Here's the drawing with two shaded views (mm, measured from the low corner). I have some questions. Coordinates: 2 decimals unless noted, no trailing zeros. Order: outer loops, then holes, each group sorted by start corner. A loop starts at its lowest first (then second) coordinate and runs counter-clockwise, first axis right, second up. Notation, with made-up numbers: (-8, -4) - (33, -4) arc R10 ccw to (33, 8) - close; hole circle Ø5 at (86.25, 27.5). An arc over 180 degrees is marked (long way). Answer as a JSON object with one key per item and string values. Group by question number.
(1) Will this pin go through, and if not, where does the flat tip stop? P1, Ø6.5, axis at x = 7.65, z = 8.87, coming from the -Y side.
(2) Imagine slicing it at A-A, the plane x = 5.5. Write out the boundary of the cut face in (y, z), and give its area (3 significant figures).
(3) Please list where these lines run through material, in increasing order: probe 1 along X at (y, z) = (11.25, 8.5); probe 2 along Z at (x, y) = (56, 10.25); probe 3 along Z at (x, y) = (7, 9.75).
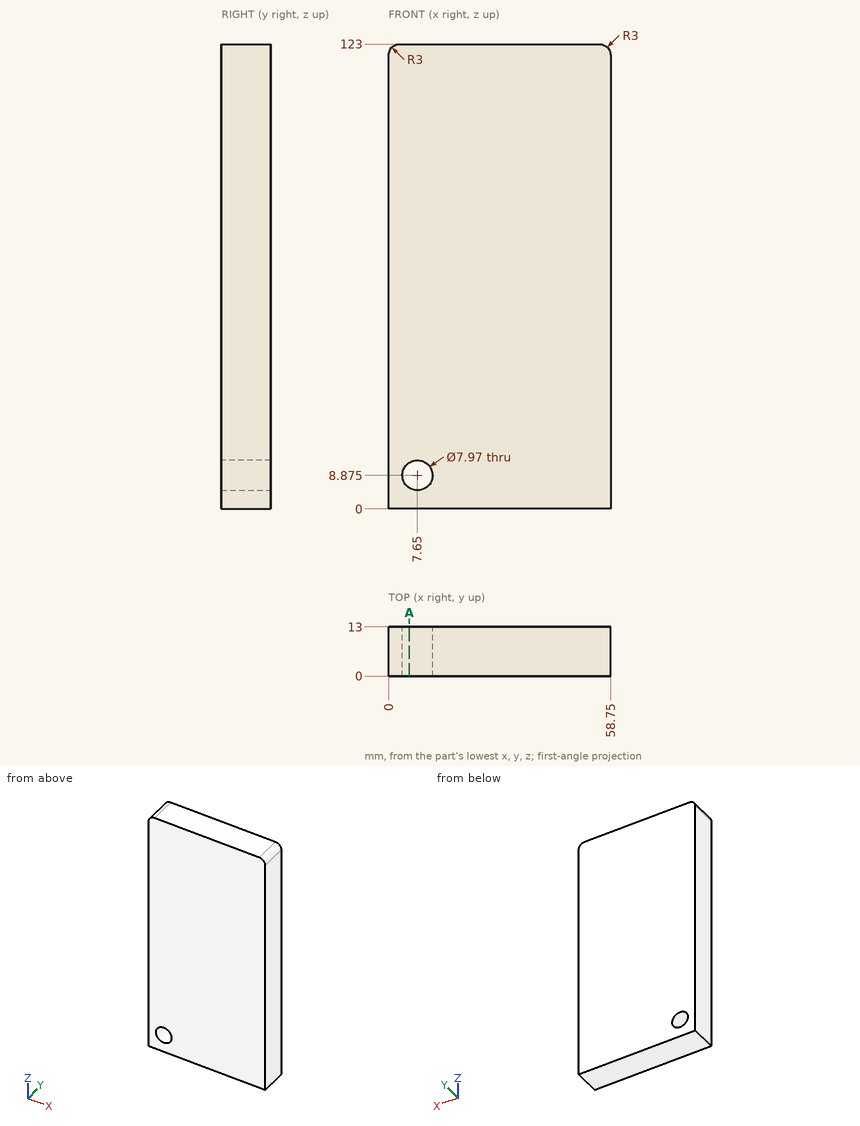
Result set:
{
 "1": {"P1": "passes through"},
 "2": {"outline": "(0, 0) - (13, 0) - (13, 5.52) - (0, 5.52) - close; (0, 12.23) - (13, 12.23) - (13, 123) - (0, 123) - close", "area": "1,510 mm^2"},
 "3": {"probe 1": "x = 0 to 3.68, 11.62 to 58.75", "probe 2": "z = 0 to 122.99", "probe 3": "z = 0 to 4.94, 12.81 to 123"}
}
